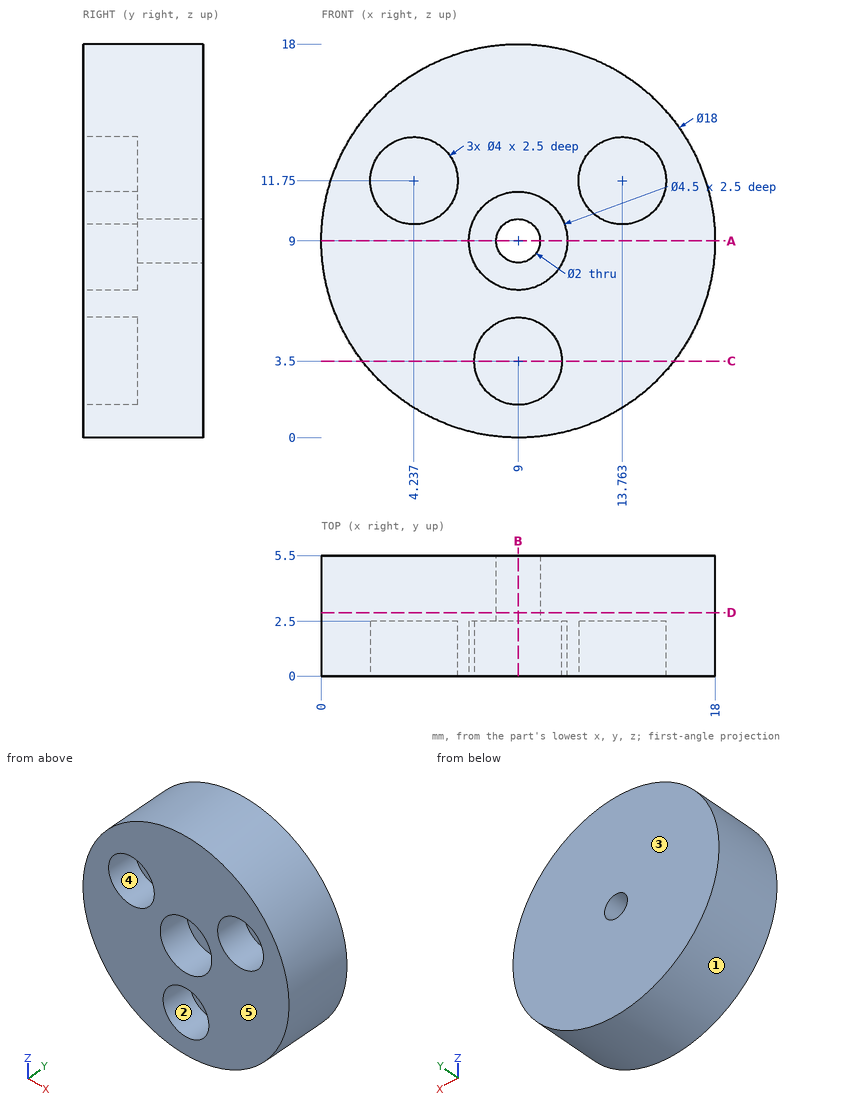
Answer from the drawing. Dimensions are ordinates in mm from the lowest x, y and z of the part. A direction names the side the tool comes from. Give positions to 0.01 mm unless a question says otherwise; leave off trailing zeros. Loops run counter-clockwise (first coordinate to the right, second up) from the corner with the lowest first, then second, coordinate; pieces in that order, holes last. Notation, with made-up numbers: (88, 60.5) -> (115, 60.5) arc R23 ccw to (115, 86.5) -> close; hole circle Ø7 at (77, -5). An arc over 180 degrees is marked (long way). Use a Markdown table: item, result.
Q1. A tool of negligible diameter and unlimited length cuts with its end or side. For the marked faces 4 and 5, from which of +Z, -Z, +X, -X, +Y, -Y can it reach the whole face along a straight path? Write none if from no direction.
Solved:
| item | result |
|---|---|
| face 4 | -Y |
| face 5 | +Z, -Z, +X, -X, -Y |
Q2. Each of these flat-tipped pins is pushed along its axis until it touches: pin 1 (1.6 mm diameter, centred on x = 9, z = 9, fed in from -Y); pin 2 (1.2 mm diameter, centred on x = 14, z = 12, fed in from -Y); pin 3 (1 mm diameter, centred on y = 3, z = 5, fed in from -X). Where does it stop, or does it pass through?
Solved:
| item | result |
|---|---|
| pin 1 | passes through |
| pin 2 | stops at y = 2.5 |
| pin 3 | stops at x = 0.71 |
Q3. Section C-C, the plane z = 3.5 is taken. Determine the outline of the cut face in (x, y).
Solved:
| item | result |
|---|---|
| outline | (1.88, 0) -> (7, 0) -> (7, 2.5) -> (11, 2.5) -> (11, 0) -> (16.12, 0) -> (16.12, 5.5) -> (1.88, 5.5) -> close |
Q4. Section B-B, the plane x = 9 is taken. Determine the outline of the cut face in (y, z).
Solved:
| item | result |
|---|---|
| outline | (0, 0) -> (5.5, 0) -> (5.5, 8) -> (2.5, 8) -> (2.5, 6.75) -> (0, 6.75) -> (0, 5.5) -> (2.5, 5.5) -> (2.5, 1.5) -> (0, 1.5) -> close; (0, 11.25) -> (2.5, 11.25) -> (2.5, 10) -> (5.5, 10) -> (5.5, 18) -> (0, 18) -> close |
Q5. Determine the mould class of the marked faces 1, 2 and 3 for opening direction X: pulls with the +X half, pulls with the -X half, needs draft (parallel to the pull), parting line crosses it, or undercut.
Solved:
| item | result |
|---|---|
| face 1 | parting line crosses it |
| face 2 | undercut |
| face 3 | needs draft |
Q6. Section A-A, the plane z = 9 is taken. Determine the outline of the cut face in (x, y).
Solved:
| item | result |
|---|---|
| outline | (0, 0) -> (6.75, 0) -> (6.75, 2.5) -> (8, 2.5) -> (8, 5.5) -> (0, 5.5) -> close; (10, 2.5) -> (11.25, 2.5) -> (11.25, 0) -> (18, 0) -> (18, 5.5) -> (10, 5.5) -> close |
Q7. Section D-D, the plane y = 2.9 is taken. Determine the outline of the cut face in (x, z).
Solved:
| item | result |
|---|---|
| outline | circle Ø18 at (9, 9); hole circle Ø2 at (9, 9) |
Q8. Find the intervals of material crossed by line 1 along Z through (x, y) = (9, 0.85); line 2 along X through (y, z) = (1.7, 13.25); line 3 along X through (y, z) = (0.85, 13) (1 decimal), in increasing order.
Solved:
| item | result |
|---|---|
| line 1 | z = 0 to 1.5, 5.5 to 6.75, 11.25 to 18 |
| line 2 | x = 1.07 to 2.91, 5.56 to 12.44, 15.09 to 16.93 |
| line 3 | x = 0.9 to 2.7, 5.8 to 12.2, 15.3 to 17.1 |
